Check sheet for the modelled part. Datum: model origin and axes. Units: mm. Face numbers are marked on the shaded views. A direction names the side the tool comes from. Coordinates: 2 decimals unless noted, no trailing zeros. Loops run counter-clockwise (first coordinate to the right, second up) from the corner with the lowest first, then second, coordinate; pieces in that order, holes last. Notation, with made-up numbers: (46.5, 21) - (105.5, 21) arc R32 ccw to (105.5, 53) - close; hole circle Ø9 at (-3.5, 31). An arc over 180 degrees is marked (long way). Use a Markdown table: item, result. Add a question column.
1) Sectioned sample at A-A, the plane z = -13.75. Enter the section's corners in (x, y), then the cut area to 3 significant figures.
2) Thickness scan on line 1 (X direction, y = 9, z = -16); line 2 (Y direction, x = -34.25, z = -19.75); line 3 (Y direction, x = -22.5, z = -1). Record the ranges inside material, lowest first.
3) Sectioned sample at C-C, the plane x = -36.25. Enter the section's corners in (y, z), then the cut area to 3 significant figures.
4) Go/stop test with flat-tipped pins: P1, Ø1.5, axis at x = -25.5, z = -3, coming from the -Y side; P2, Ø0.8, axis at y = 8.5, z = -17, coming from the +X side; P3, Ø1.5, axis at y = 7.5, z = -11, coming from the -X side; P4, Ø1.9, axis at x = -14, z = -11.5, coming from the +Y side. Record where each tip stops, or that it passes through.
5) Tool access check on the marked faces 1, 2 and 3. Record the directions out of +Z, -Z, +X, -X, +Y, -Y that give a thin tool (end or side, any length) a straight path to the whole face; none if there is none.
6) Sectioned sample at B-B, the plane y = 10.5. Enter the section's corners in (x, z).
7) Sectioned sample at D-D, the plane y = 6.75. Enter the section's corners in (x, z), then the cut area to 3 significant figures.
Autodesk Fusion 360 part; units mm, degrees
sketch "Sketch1" plane through (0, 0, 0) normal (0, 1, 0) x (1, 0, 0)
  line L0 (-40.1743, 28.9794) -> (-10.1743, 28.9794)
  line L1 (-10.1743, 28.9794) -> (-10.1743, -1.0206)
  line L2 (-10.1743, -1.0206) -> (-40.1743, -1.0206)
  line L3 (-40.1743, -1.0206) -> (-40.1743, 28.9794)
  dimension "d1" = 30
  dimension "d2" = 30
extrude "Extrude1" add sketch "Sketch1" along normal blind 5
sketch "Sketch2" plane through (0, 0, 1.0206) normal (0, 0, 1) x (1, 0, 0)
  line L0 (-40.1743, 0) -> (-10.1743, 0)
  line L1 (-10.1743, 0) -> (-10.1743, 5)
  line L2 (-10.1743, 5) -> (-40.1743, 5)
  line L3 (-40.1743, 5) -> (-40.1743, 0)
  circle A0 centre (-25.1743, 9) radius 4
  circle A1 centre (-25.1743, 9) radius 5.5
  line L4 (-19.6743, 9) -> (-19.6743, 5)
  line L5 (-30.6743, 9) -> (-30.6743, 4.9999)
  dimension "d8" = 8
  dimension "d9" = 11
extrude "Extrude2" add sketch "Sketch2" against normal blind 30 contours L2 A1 L5 | L2 A1 L4 | L2 A1 picked at (-30.1523, 9.3387)
fillet "Fillet1" radius 3 2 edges at (-19.6743, 5, -13.9794) (-30.6743, 5, -13.9794)
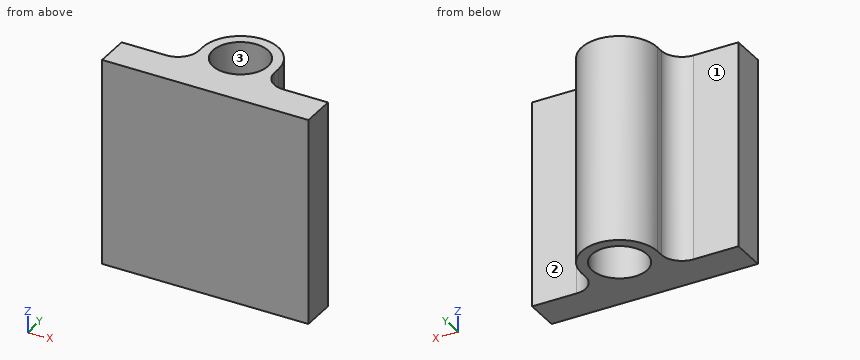
Solved:
| question | item | result |
|---|---|---|
| 1 | outline | (-40.17, 0) - (-10.17, 0) - (-10.17, 5) - (-16.67, 5) arc R3 cw to (-19.67, 8) - (-19.67, 9) arc R5.5 ccw to (-30.67, 9) - (-30.67, 8) arc R3 cw to (-33.67, 5) - (-40.17, 5) - close; hole circle Ø8 at (-25.17, 9) |
| 1 | area | 195 mm2 |
| 2 | line 1 | x = -30.67 to -29.17, -21.17 to -19.67 |
| 2 | line 2 | y = 0 to 5 |
| 2 | line 3 | y = 0 to 6.03, 11.97 to 13.81 |
| 3 | outline | (0, -28.98) - (5, -28.98) - (5, 1.02) - (0, 1.02) - close |
| 3 | area | 150 mm2 |
| 4 | P1 | stops at y = 0 |
| 4 | P2 | stops at x = -19.67 |
| 4 | P3 | stops at x = -30.95 |
| 4 | P4 | stops at y = 5 |
| 5 | face 1 | +Z, -Z, -X, +Y |
| 5 | face 2 | +Z, -Z, +X, +Y |
| 5 | face 3 | +Z, -Z |
| 6 | outline | (-30.47, -28.98) - (-28.88, -28.98) - (-28.88, 1.02) - (-30.47, 1.02) - close; (-21.47, -28.98) - (-19.88, -28.98) - (-19.88, 1.02) - (-21.47, 1.02) - close |
| 7 | outline | (-30.95, -28.98) - (-28.48, -28.98) - (-28.48, 1.02) - (-30.95, 1.02) - close; (-21.87, -28.98) - (-19.4, -28.98) - (-19.4, 1.02) - (-21.87, 1.02) - close |
| 7 | area | 148 mm2 |
